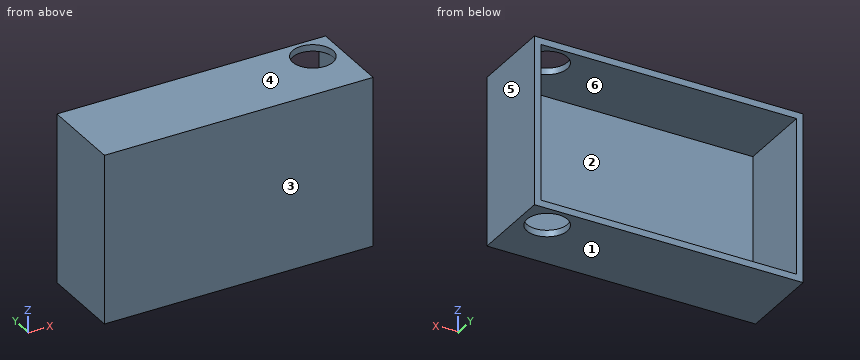
from build123d import *

# Parameters (mm, degrees)
SKETCH1_W           = 787.4
SKETCH1_H           = 495.3
BOSS_EXTRUDE1_DEPTH = 241.3
SHELL1_T            = -19.05
SKETCH2_R           = 59.309
CUT_EXTRUDE1_DEPTH  = 496.3


with BuildPart() as part:
    # Sketch1 → Boss-Extrude1 (new body)
    with BuildSketch(Plane(origin=(0, 0, 0), x_dir=(1, 0, 0), z_dir=(0, 1, 0))):
        with Locations((393.7, 247.65)):
            Rectangle(SKETCH1_W, SKETCH1_H)
    extrude(amount=BOSS_EXTRUDE1_DEPTH)

    # Shell1
    shell1_openings = [part.faces().sort_by_distance(p)[0] for p in [
        (393.7, 241.3, -247.65),
    ]]
    offset(amount=SHELL1_T, openings=shell1_openings, kind=Kind.INTERSECTION)

    # Sketch2 → Cut-Extrude1 (cut, through all)
    with BuildSketch(Plane.XY):
        with Locations((708.025, 168.275)):
            Circle(SKETCH2_R)
    extrude(amount=-CUT_EXTRUDE1_DEPTH, mode=Mode.SUBTRACT)


solid = part.part
Here's how the part is built. I have some questions about the finished solid (model axes, mm). Face numbers are marked on the shaded views. A direction names the side the tool comes from. Round coordinates to 2 decimals unless told otherwise and drop trailing zeros. Loops run counter-clockwise (first coordinate to the right, second up) from the corner with the lowest first, then second, coordinate; pieces in that order, holes last. Notation, with made-up numbers: (25.5, -21) -> (44.5, -21) arc R28 ccw to (44.5, 9) -> close; hole circle Ø4 at (45, -40). An arc over 180 degrees is marked (long way). Write each question's results on one line, items separated by ' | '.
(1) If we section it at C-C, the plane y = 37: List the corners of the cut face in (x, z) for me.
Worked answers:
outline: (0, -495.3) -> (787.4, -495.3) -> (787.4, 0) -> (0, 0) -> close; hole (19.05, -476.25) -> (768.35, -476.25) -> (768.35, -19.05) -> (19.05, -19.05) -> close
(2) For the marked faces 5 and 6, which set-ups out of +Z, -Z, +X, -X, +Y, -Y let a thin tool reach every point of the face, with its end or its side?
Worked answers:
face 5: +Z, -Z, +X, +Y, -Y | face 6: +Y
(3) If we section it at A-A, the plane z = -75.5: List the corners of the cut face in (x, y) for me.
Worked answers:
outline: (0, 0) -> (787.4, 0) -> (787.4, 241.3) -> (768.35, 241.3) -> (768.35, 19.05) -> (19.05, 19.05) -> (19.05, 241.3) -> (0, 241.3) -> close
(4) For P1, Ø5, axis at x = 632.5, z = -378.5, coming from the +Y side, with a flat end and sliding along its axis, tell me the tip position at first contact or that it passes through.
Worked answers:
P1: y = 19.05
(5) If we section it at B-B, the plane x = 690: List the corners of the cut face in (y, z) for me, then the cut area to 3 significant figures.
Worked answers:
outline: (0, -495.3) -> (111.77, -495.3) -> (111.77, -476.25) -> (19.05, -476.25) -> (19.05, -19.05) -> (111.77, -19.05) -> (111.77, 0) -> (0, 0) -> close; (224.78, -495.3) -> (241.3, -495.3) -> (241.3, -476.25) -> (224.78, -476.25) -> close; (224.78, -19.05) -> (241.3, -19.05) -> (241.3, 0) -> (224.78, 0) -> close | area: 13,600 mm2
(6) We'd pull the mould along Z, two halves only. Please class the marked faces 1, 2, 3 and 4: released by +Z, released by -Z, zero draft, split by the parting line, or undercut.
Worked answers:
face 1: released by -Z | face 2: undercut | face 3: zero draft | face 4: released by +Z
(7) If we section it at D-D, the plane y = 181: List the corners of the cut face in (x, z) for me, then the cut area to 3 significant figures.
Worked answers:
outline: (0, -495.3) -> (650.1, -495.3) -> (650.1, -476.25) -> (19.05, -476.25) -> (19.05, -19.05) -> (650.1, -19.05) -> (650.1, 0) -> (0, 0) -> close; (765.95, -495.3) -> (787.4, -495.3) -> (787.4, 0) -> (765.95, 0) -> (765.95, -19.05) -> (768.35, -19.05) -> (768.35, -476.25) -> (765.95, -476.25) -> close | area: 43,000 mm2
(8) If I drill on L1, parallel to X at y = 73.5, z = -274; L2, parallel to Z at x = 649, y = 129.5, over which ranges is the centre line in solid material (lowest first)?
Worked answers:
L1: 0 to 19.05, 768.35 to 787.4 | L2: -495.3 to -476.25, -19.05 to 0
